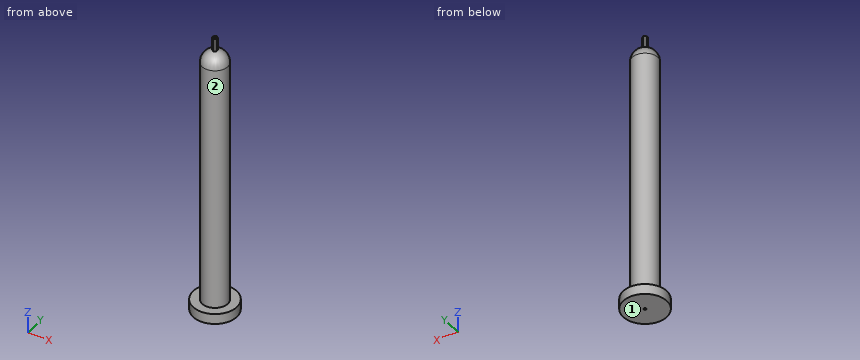
```python
from build123d import *

# Parameters (mm, degrees)
F0_R      = 8.5
F1_DEPTH  = 4
F2_R      = 5
F3_DEPTH  = 100
F9_DEPTH  = 5
F10_R     = 0.5
F11_DEPTH = 117.5


with BuildPart() as f1:
    # F0 (on Top) → F1 (new body)
    with BuildSketch(Plane.XY):
        Circle(F0_R)
    extrude(amount=F1_DEPTH)

    # F2 (on Top) → F3 (join)
    with BuildSketch(Plane.XY):
        Circle(F2_R)
    extrude(amount=F3_DEPTH)

    # F4 (on Right) → F6 (revolve)
    with BuildSketch(Plane.YZ):
        with BuildLine():
            Line((0, 104.898979), (0, 100))
            Line((0, 100), (5, 100))
            ThreePointArc((5, 100), (3.872983, 103.162278), (1, 104.898979))
            Line((1, 104.898979), (0, 104.898979))
        make_face()
    revolve(axis=Axis((0, 0, 102.5), (0, 0, -1)))

    # F8 (on face) → F9 (join)
    with BuildSketch(Plane(origin=(0, 0, 104.898979), x_dir=(1, 0, 0), z_dir=(0, 0, -1))):
        Polygon((0.866025, -0.5), (0.866025, 0.5), (0, 1), (-0.866025, 0.5), (-0.866025, -0.5), (0, -1), align=None)
    extrude(amount=-F9_DEPTH)

    # F10 (on face) → F11 (cut)
    with BuildSketch(Plane(origin=(0, 0, 0), x_dir=(1, 0, 0), z_dir=(0, 0, -1))):
        Circle(F10_R)
    extrude(amount=-F11_DEPTH, mode=Mode.SUBTRACT)


solid = f1.part
```
Design review of the part built by this model. Coordinates are the model's own, in mm. Face numbers are marked on the shaded views. A direction names the side the tool comes from. Coordinates: 2 decimals unless noted, no trailing zeros. Order: outer loops, then holes, each group sorted by start corner. A loop starts at its lowest first (then second) coordinate and runs counter-clockwise, first axis right, second up.
1) Take a section at A-A, the plane z = 39. Give the boundary of the cut face in (x, y), and give its area (3 significant figures).
2) Wall thickness on line 1 along X through (y, z) = (0, 65.5); line 2 along Z through (x, y) = (-7, 1.25): over which ranges is each line inside the solid? List them lowest first.
3) Clearance check with flat-ended pins moving along their axes: pin 1 (1 mm diameter, centred on x = 6, y = 1.5, fed in from +Z); pin 2 (10 mm diameter, centred on x = 4, z = 34, fed in from +Y); pin 3 (5 mm diameter, centred on x = -2.5, y = -5.5, fed in from +Z). State where each tip first meets the part, or that it passes through.
4) For the marked faces 1 and 2, list the 3-axis set-ups (+Z, -Z, +X, -X, +Y, -Y) from which the entire face can be reached by the end or side of a thin tool; tool diameter is ignored.
5) Take a section at B-B, the plane x = 7. Give the boundary of the cut face in (y, z), and give its area (3 significant figures).
Returned:
1. outline: circle Ø10 at (0, 0); hole circle Ø1 at (0, 0)
1. area: 77.8 mm2
2. line 1: x = -5 to -0.5, 0.5 to 5
2. line 2: z = 0 to 4
3. pin 1: stops at z = 4
3. pin 2: stops at y = 5
3. pin 3: stops at z = 103.53
4. face 1: -Z, +X, -X, +Y, -Y
4. face 2: +Z
5. outline: (-4.82, 0) - (4.82, 0) - (4.82, 4) - (-4.82, 4) - close
5. area: 38.6 mm2
